Autodesk Inventor part; units mm, degrees
ref_plane "YZ Plane" through (0, 0, 0) normal (1, 0, 0) x (0, 1, 0)
ref_plane "XZ Plane" through (0, 0, 0) normal (0, 1, 0) x (-1, 0, 0)
ref_plane "XY Plane" through (0, 0, 0) normal (0, 0, 1) x (1, 0, 0)
sketch "Sketch2" plane through (0, 0, 0) normal (0, 1, 0) x (-1, 0, 0)
  line L0 (-89, 99) -> (89, 99)
  line L1 (89, 99) -> (89, -99)
  line L2 (89, -99) -> (-89, -99)
  line L3 (-89, -99) -> (-89, 99)
  line L4 (-89, 99) -> (89, -99) construction
  line L5 (89, 99) -> (-89, -99) construction
  line L6 (-89, 99) -> (89, 99)
  line L7 (89, 99) -> (89, -85)
  line L8 (89, -85) -> (-89, -85)
  line L9 (-89, -85) -> (-89, 99)
  line L10 (-4.5, 99) -> (-89, 99)
  line L11 (-89, 99) -> (-89, 46)
  line L12 (-89, 46) -> (-4.5, 46)
  line L13 (-4.5, 46) -> (-4.5, 99)
  line L14 (4.5, 99) -> (89, 99)
  line L15 (89, 99) -> (89, 46)
  line L16 (89, 46) -> (4.5, 46)
  line L17 (4.5, 46) -> (4.5, 99)
  line L18 (22.5, 77.5) -> (22.5, 66.5)
  line L19 (16.5, 66.5) -> (16.5, 77.5)
  line L20 (-22.5, 66.5) -> (-22.5, 77.5)
  line L21 (-16.5, 77.5) -> (-16.5, 66.5)
  line L22 (-22.5, 99) -> (-16.5, 99)
  line L23 (-16.5, 99) -> (-16.5, 46)
  line L24 (-16.5, 46) -> (-22.5, 46)
  line L25 (-22.5, 46) -> (-22.5, 99)
  line L26 (16.5, 99) -> (22.5, 99)
  line L27 (22.5, 99) -> (22.5, 46)
  line L28 (22.5, 46) -> (16.5, 46)
  line L29 (16.5, 46) -> (16.5, 99)
  line L30 (-89, 99) -> (89, 99)
  line L31 (89, 99) -> (89, 98)
  line L32 (89, 98) -> (-89, 98)
  line L33 (-89, 98) -> (-89, 99)
  point P0 (0, 0)
  point P1 (4.5, 99)
  point P2 (-4.5, 99)
  point P3 (-89, 46)
  point P4 (89, 46)
  point P5 (4.5, 98)
  point P6 (-4.5, 98)
  point P7 (-16.5, 98)
  point P8 (-22.5, 98)
  point P9 (22.5, 98)
  point P10 (16.5, 98)
  dimension "d8" = 178
  dimension "d9" = 198
  dimension "d10" = 14
  dimension "d11" = 84.5
  dimension "d12" = 53
  dimension "d13" = 84.5
  dimension "d14" = 53
  dimension "d17" = 9
  dimension "d18" = 1
extrude "Extrusion2" add sketch "Sketch2" along normal blind 3 contours L32 L23 L21 L12 L25 L20 | L12 L13 L32 L17 L16 L1 L8 L3 | L32 L27 L18 L16 L29 L19
equation "\"d11\" = d13"
properties part number "base" material "Steel, Alloy"
Work out the finished part from the listing and answer in its coordinate system (mm). Coordinates: 2 decimals unless noted, no trailing zeros. Write each loop counter-clockwise with the first axis right and the second up, starting at its lowest first coordinate (ties: lowest second). Pieces come first, ordered by that corner, then holes.
Q1. A cutting plane is placed at B-B, the plane y = 1.85. Give the vertices of the cut face in (x, z).
Q2. A cutting plane is placed at C-C, the plane x = 10. Give the vertices of the cut face in (y, z), then the cut area to 3 significant figures.
Q3. Find the intervals of material crossed by line 1 (X direction, y = 2.3, z = 53); line 2 (Z direction, x = 46.5, y = 2), in increasing order.
Q4. Each of these flat-tipped pins is pushed along its axis until it touches: pin 1 Ø1.5 at (x, y) = (-10, 2) entering from +Z; pin 2 Ø0.9 at (y, z) = (1, 63.5) entering from +X; pin 3 Ø1 at (x, z) = (22.5, -56) entering from -Y; pin 4 Ø0.9 at (y, z) = (1.5, 72) entering from -X. Where does it stop, or does it pass through?
Q5. A cutting plane is placed at A-A, the plane z = 79.5. Give the vertices of the cut face in (x, y).
Findings below:
1. outline: (-89, -85) - (89, -85) - (89, 46) - (22.5, 46) - (22.5, 98) - (16.5, 98) - (16.5, 46) - (4.5, 46) - (4.5, 98) - (-4.5, 98) - (-4.5, 46) - (-16.5, 46) - (-16.5, 98) - (-22.5, 98) - (-22.5, 46) - (-89, 46) - close
2. outline: (0, -85) - (3, -85) - (3, 46) - (0, 46) - close
2. area: 393 mm2
3. line 1: x = -22.5 to -16.5, -4.5 to 4.5, 16.5 to 22.5
3. line 2: z = -85 to 46
4. pin 1: stops at z = 46
4. pin 2: stops at x = 22.5
4. pin 3: stops at y = 0
4. pin 4: stops at x = -22.5
5. outline: (-22.5, 0) - (-16.5, 0) - (-16.5, 3) - (-22.5, 3) - close; (-4.5, 0) - (4.5, 0) - (4.5, 3) - (-4.5, 3) - close; (16.5, 0) - (22.5, 0) - (22.5, 3) - (16.5, 3) - close
